Autodesk Inventor part; units mm, degrees
ref_plane "YZ Plane" through (0, 0, 0) normal (1, 0, 0) x (0, 1, 0)
ref_plane "XZ Plane" through (0, 0, 0) normal (0, 1, 0) x (-1, 0, 0)
ref_plane "XY Plane" through (0, 0, 0) normal (0, 0, 1) x (1, 0, 0)
sketch "Sketch1" plane through (0, 0, 0) normal (0, 0, 1) x (1, 0, 0)
  line L0 (0, 0) -> (-128, 0)
  line L1 (-128, 87.5) -> (0, 87.5)
  line L2 (0, 87.5) -> (0, 0)
  line L3 (-128, 71.5) -> (-138, 61.5)
  line L4 (-138, 61.5) -> (-138, 19.5)
  line L5 (-138, 19.5) -> (-128, 9.5)
  line L6 (-128, 0) -> (-128, 9.5)
  line L7 (-128, 71.5) -> (-128, 87.5)
  line L8 (-52, 9.5) -> (-44, 9.5)
  line L9 (-44, 9.5) -> (-44, 3)
  line L10 (-44, 3) -> (-52, 3)
  line L11 (-52, 3) -> (-52, 9.5)
  line L12 (-52, 78) -> (-44, 78)
  line L13 (-44, 78) -> (-44, 71.5)
  line L14 (-44, 71.5) -> (-52, 71.5)
  line L15 (-52, 71.5) -> (-52, 78)
  line L16 (-16, 78) -> (-8, 78)
  line L17 (-8, 78) -> (-8, 71.5)
  line L18 (-8, 71.5) -> (-16, 71.5)
  line L19 (-16, 71.5) -> (-16, 78)
  line L20 (-16, 9.5) -> (-8, 9.5)
  line L21 (-8, 9.5) -> (-8, 3)
  line L22 (-8, 3) -> (-16, 3)
  line L23 (-16, 3) -> (-16, 9.5)
  line L24 (-34, 84.5) -> (-26, 84.5)
  line L25 (-26, 84.5) -> (-26, 78)
  line L26 (-26, 78) -> (-34, 78)
  line L27 (-34, 78) -> (-34, 84.5)
  line L28 (-6, 50.4411) -> (-6, 30.5589)
  line L29 (-6, 30.5589) -> (-20.0589, 16.5)
  line L30 (-20.0589, 16.5) -> (-39.9411, 16.5)
  line L31 (-39.9411, 16.5) -> (-54, 30.5589)
  line L32 (-54, 30.5589) -> (-54, 50.4411)
  line L33 (-54, 50.4411) -> (-39.9411, 64.5)
  line L34 (-39.9411, 64.5) -> (-20.0589, 64.5)
  line L35 (-20.0589, 64.5) -> (-6, 50.4411)
  line L36 (-51, 61.5) -> (-9, 61.5) construction
  line L37 (-9, 61.5) -> (-9, 19.5) construction
  line L38 (-9, 19.5) -> (-51, 19.5) construction
  line L39 (-51, 19.5) -> (-51, 61.5) construction
  circle A0 centre (-51, 61.5) radius 3.2
  circle A1 centre (-51, 19.5) radius 3.2
  circle A2 centre (-9, 19.5) radius 3.2
  circle A3 centre (-9, 61.5) radius 3.2
  circle A4 centre (-131, 60.5) radius 2.75
  circle A5 centre (-131, 20.5) radius 2.75
  line L40 (-124, 78) -> (-116, 78)
  line L41 (-116, 78) -> (-116, 71.5)
  line L42 (-116, 71.5) -> (-124, 71.5)
  line L43 (-124, 71.5) -> (-124, 78)
  line L44 (-124, 9.5) -> (-116, 9.5)
  line L45 (-116, 9.5) -> (-116, 3)
  line L46 (-116, 3) -> (-124, 3)
  line L47 (-124, 3) -> (-124, 9.5)
  line L48 (-121, 63.5) -> (-113, 63.5)
  line L49 (-113, 63.5) -> (-113, 57)
  line L50 (-113, 57) -> (-121, 57)
  line L51 (-121, 57) -> (-121, 63.5)
  line L52 (-121, 24) -> (-113, 24)
  line L53 (-113, 24) -> (-113, 17.5)
  line L54 (-113, 17.5) -> (-121, 17.5)
  line L55 (-121, 17.5) -> (-121, 24)
  circle A6 centre (-66, 67.5) radius 2.75
  circle A7 centre (-66, 13.5) radius 2.75
  line L56 (-60, 87.5) -> (-60, 0) construction
  line L57 (-132, 67.5) -> (-60, 67.5) construction
  line L58 (-132, 13.5) -> (-60, 13.5) construction
  line L59 (-83, 63.5) -> (-75, 63.5)
  line L60 (-75, 63.5) -> (-75, 57)
  line L61 (-75, 57) -> (-83, 57)
  line L62 (-83, 57) -> (-83, 63.5)
  line L63 (-83, 24) -> (-75, 24)
  line L64 (-75, 24) -> (-75, 17.5)
  line L65 (-75, 17.5) -> (-83, 17.5)
  line L66 (-83, 17.5) -> (-83, 24)
  line L67 (-73, 78) -> (-65, 78)
  line L68 (-65, 78) -> (-65, 71.5)
  line L69 (-65, 71.5) -> (-73, 71.5)
  line L70 (-73, 71.5) -> (-73, 78)
  line L71 (-73, 9.5) -> (-65, 9.5)
  line L72 (-65, 9.5) -> (-65, 3)
  line L73 (-65, 3) -> (-73, 3)
  line L74 (-73, 3) -> (-73, 9.5)
  line L75 (-113, 84.5) -> (-105, 84.5)
  line L76 (-105, 84.5) -> (-105, 78)
  line L77 (-105, 78) -> (-113, 78)
  line L78 (-113, 78) -> (-113, 84.5)
  line L79 (-84, 84.5) -> (-76, 84.5)
  line L80 (-76, 84.5) -> (-76, 78)
  line L81 (-76, 78) -> (-84, 78)
  line L82 (-84, 78) -> (-84, 84.5)
  circle A8 centre (-106, 40.5) radius 2.75
  circle A9 centre (-74, 40.5) radius 2.75
  point P0 (-30, 40.5)
  point P1 (-138, 40.5)
  point P2 (-54, 40.5)
  point P3 (-51, 40.5)
  point P4 (-30, 61.5)
  point P5 (-30, 64.5)
  dimension "d1" = 45
  dimension "d2" = 10
  dimension "d5" = 3
  dimension "d6" = 8
  dimension "d7" = 8
  dimension "d8" = 6.5
  dimension "d10" = 3
  dimension "d11" = 48
  dimension "d12" = 8
  dimension "d13" = 6
  dimension "d14" = 42
  dimension "d15" = 42
  dimension "d16" = 6.4
  dimension "d17" = 6.4
  dimension "d18" = 6.4
  dimension "d19" = 6.4
  dimension "d20" = 5.5
  dimension "d21" = 5.5
  dimension "d22" = 7
  dimension "d23" = 11
  dimension "d24" = 11
  dimension "d25" = 6.5
  dimension "d26" = 8
  dimension "d27" = 6.5
  dimension "d28" = 6.5
  dimension "d29" = 8
  dimension "d30" = 6.5
  dimension "d31" = 8
  dimension "d32" = 8
  dimension "d33" = 5.5
  dimension "d34" = 5.5
  dimension "d35" = 4
  dimension "d36" = 4
  dimension "d37" = 8
  dimension "d38" = 8
  dimension "d39" = 8
  dimension "d40" = 4
  dimension "d41" = 8
  dimension "d42" = 128
  dimension "d43" = 68
  dimension "d44" = 8
  dimension "d45" = 43
  dimension "d47" = 10
  dimension "d48" = 15
  dimension "d49" = 62
  dimension "d50" = 10
  dimension "d52" = 8
  dimension "d53" = 3
  dimension "d54" = 8
  dimension "d55" = 3
  dimension "d56" = 5.5
  dimension "d57" = 5.5
  dimension "d58" = 14
  dimension "d59" = 32
  dimension "d66" = 54
extrude "Extrusion1" add sketch "Sketch1" along normal blind 6.5
chamfer "Chamfer1" distance 2 angle 45 4 edges at (-128, 0, 3.25) (-128, 87.5, 3.25) (0, 87.5, 3.25) (0, 0, 3.25)
properties part number "x_iddler_bottom" material "Plywood, Finish"
Could you check a few things on this model? Use its own coordinates, in mm. Round coordinates to 2 decimals unless told otherwise and drop trailing zeros. Order: outer loops, then holes, each group sorted by start corner. A loop starts at its lowest first (then second) coordinate and runs counter-clockwise, first axis right, second up. Notation, with made-up numbers: M 69,62.5 L 109,62.5 A22 cw 109,82.5 Z; hole C -38,-30 d2. An arc over 180 degrees is marked long. One line per question, with ' | ' between items. Start each with the question number.
(1) For P1, Ø3, axis at y = 61.5, z = 3.5, coming from the +X side; P2, Ø2, axis at y = 5.5, z = 4.5, coming from the -X side, each with a flat end and sliding along its axis, tell me the tip position at first contact or that it passes through.
(2) Suppose I cut it at A-A on y = 13.5. List the corners of the cut face in (x, z) for me, then the cut area to 3 significant figures.
(3) Please list where these lines run through material, in increasing order: line 1 along Y through (x, z) = (-82, 2.75); line 2 along X through (y, z) = (77.5, 3); line 3 along X through (y, z) = (32, 1.25).
(4) Suppose I cut it at C-C on z = 2.5. Count the separate pieces of the cut face and the enclosed holes in it, then the cut area to 3 significant figures.
(5) Suppose I cut it at B-B on x = -107. List the corners of the cut face in (y, z) for me.
(6) Thinking about a two-plate mould opening in X: for faces 1 (the face through (-85, 44, 0)), 2 (the face through (-116, 75, 3)), which applies, +X half, -X half, draft (parallel to the pull), parting line (faces both ways), or undercut?
Geometry results:
1) P1: x = 0 | P2: x = -128
2) outline: M -132,0 L -68.75,0 L -68.75,6.5 L -132,6.5 Z; M -63.25,0 L 0,0 L 0,6.5 L -63.25,6.5 Z | area: 822 mm²
3) line 1: 0 to 17.5, 24 to 57, 63.5 to 78, 84.5 to 87.5 | line 2: -128 to -124, -116 to -73, -65 to -52, -44 to -16, -8 to 0 | line 3: -138 to -54, -6 to 0
4) separate pieces: 1 | enclosed holes: 26 | area: 8,750 mm²
5) outline: M 0,0 L 37.94,0 L 37.94,6.5 L 0,6.5 Z; M 43.06,0 L 78,0 L 78,6.5 L 43.06,6.5 Z; M 84.5,0 L 87.5,0 L 87.5,6.5 L 84.5,6.5 Z
6) face 1: draft | face 2: undercut
